from build123d import *

# Parameters (mm, degrees)
SKETCH1_W           = 40
SKETCH1_H           = 16
BOSS_EXTRUDE1_DEPTH = 1.5
SKETCH2_R           = 1.7
CUT_EXTRUDE1_DEPTH  = 22.592822882
SKETCH3_W           = 0.9
SKETCH3_H           = 0.4
CUT_EXTRUDE2_DEPTH  = 22.592822882
SKETCH5_R           = 1.65
CUT_EXTRUDE4_DEPTH  = 22.592822882
CUT_EXTRUDE5_DEPTH  = 0.05


with BuildPart() as part:
    # Sketch1 → Boss-Extrude1 (new body)
    with BuildSketch(Plane(origin=(0, 0, 0), x_dir=(1, 0, 0), z_dir=(0, 1, 0))):
        Rectangle(SKETCH1_W, SKETCH1_H)
    extrude(amount=BOSS_EXTRUDE1_DEPTH)

    # Sketch2 → Cut-Extrude1 (cut, through all)
    with BuildSketch(Plane(origin=(0, 1.5, 0), x_dir=(1, 0, 0), z_dir=(0, 1, 0))):
        with Locations(Location((0, 5.5, 0), (0, 0, 270))):
            Circle(SKETCH2_R)
        with Locations(Location((17.5, 5.5, 0), (0, 0, 270))):
            Circle(SKETCH2_R)
    extrude(amount=-CUT_EXTRUDE1_DEPTH, mode=Mode.SUBTRACT)

    # Sketch3 → Cut-Extrude2 (cut, through all)
    with BuildSketch(Plane(origin=(0, 1.5, 0), x_dir=(1, 0, 0), z_dir=(0, 1, 0))):
        with Locations((15.35, 1.3)):
            Rectangle(SKETCH3_W, SKETCH3_H)
        with Locations((5.15, 1.3)):
            Rectangle(SKETCH3_W, SKETCH3_H)
        with Locations((10.25, 1.3)):
            Rectangle(SKETCH3_W, SKETCH3_H)
    extrude(amount=-CUT_EXTRUDE2_DEPTH, mode=Mode.SUBTRACT)

    # Sketch5 → Cut-Extrude4 (cut, through all)
    with BuildSketch(Plane(origin=(0, 1.5, 0), x_dir=(1, 0, 0), z_dir=(0, 1, 0))):
        with Locations(Location((-15.78, 3.87, 0), (0, 0, 270))):
            Circle(SKETCH5_R)
        with Locations(Location((-15.78, -3.87, 0), (0, 0, 270))):
            Circle(SKETCH5_R)
    extrude(amount=-CUT_EXTRUDE4_DEPTH, mode=Mode.SUBTRACT)

    # Sketch6 → Cut-Extrude5 (cut)
    with BuildSketch(Plane(origin=(0, 1.5, 0), x_dir=(1, 0, 0), z_dir=(0, 1, 0))):
        Polygon((4.9, 1.5), (4.9, 2), (0.5208, 2), (0.5208, -2.8575), (-5.9792, -2.8575), (-5.9792, -2.2225), (-0.1192, -2.2225), (-0.1192, 2.5), (5.4, 2.5), (5.4, 1.5), align=None)
        Polygon((-5.9792, 2.8575), (-5.9792, 2.2225), (-0.4792, 2.2225), (-0.4792, 3), (15.1, 3), (15.1, 1.5), (15.6, 1.5), (15.6, 3.5), (-1.1192, 3.5), (-1.1192, 2.8575), align=None)
    extrude(amount=-CUT_EXTRUDE5_DEPTH, mode=Mode.SUBTRACT)


solid = part.part
Part model, mm, in its own coordinate system. A direction names the side the tool comes from. Round coordinates to 2 decimals unless told otherwise and drop trailing zeros. Write each loop counter-clockwise with the first axis right and the second up, starting at its lowest first coordinate (ties: lowest second). Pieces come first, ordered by that corner, then holes. Notation, with made-up numbers: M 59.5,-8.5 L 82.5,-8.5 A31 cw 82.5,30.5 Z; hole C 46.25,-23.75 d3. An arc over 180 degrees is marked long. Return JSON: item names as keys, results as strings. Group by question number.
(1) Two-plate mould, pull along X, no slides. Class faces 1 (the face through (0, 1, 8)), 2 (the face through (15.3, 0.8, -1.1)), 3 (the face through (-20, 1, 0)): +X half, -X half, draft (parallel to the pull), parting line (faces both ways), or undercut.
(2) Which spindle directions (+Z, -Z, +X, -X, +Y, -Y) get a long thin tool onto all of the face, cutting with end or side? Do faces 4 (the face through (5, 1, -1.5)), 5 (the face through (20, 1, 0)). Say none if no direction does.
(3) Saw through at B-B on y = 0.35. Write the cut outline in (x, z), then the cut area to 3 significant figures.
(4) Saw through at A-A on x = 17.5. Write the cut outline in (y, z).
(5) Saw through at D-D on x = -15.78. Write the cut outline in (y, z), then the cut area to 3 significant figures.
(6) Drill centre lines: probe 1 along X at (y, z) = (0.6, 3.75); probe 2 along X at (y, z) = (0.9, -4); probe 3 along Z at (x, y) = (17, 0.5). Where is each one in solid material? Low to high.
(7) Saw through at C-C on z = 3.87. Write the cut outline in (x, y), then the cut area to 4 significant figures.
Returned:
{
 "1": {"face 1": "draft", "face 2": "undercut", "face 3": "-X half"},
 "2": {"face 4": "+Y, -Y", "face 5": "+Z, -Z, +X, +Y, -Y"},
 "3": {"outline": "M -20,-8 L 20,-8 L 20,8 L -20,8 Z; hole C -15.78,-3.87 d3.3; hole C -15.78,3.87 d3.3; hole C 0,-5.5 d3.4; hole M 4.7,-1.5 L 5.6,-1.5 L 5.6,-1.1 L 4.7,-1.1 Z; hole M 9.8,-1.5 L 10.7,-1.5 L 10.7,-1.1 L 9.8,-1.1 Z; hole M 14.9,-1.5 L 15.8,-1.5 L 15.8,-1.1 L 14.9,-1.1 Z; hole C 17.5,-5.5 d3.4", "area": "604 mm²"},
 "4": {"outline": "M 0,-8 L 1.5,-8 L 1.5,-7.2 L 0,-7.2 Z; M 0,-3.8 L 1.5,-3.8 L 1.5,8 L 0,8 Z"},
 "5": {"outline": "M 0,-8 L 1.5,-8 L 1.5,-5.52 L 0,-5.52 Z; M 0,-2.22 L 1.5,-2.22 L 1.5,2.22 L 0,2.22 Z; M 0,5.52 L 1.5,5.52 L 1.5,8 L 0,8 Z", "area": "14.1 mm²"},
 "6": {"probe 1": "-20 to -17.43, -14.13 to 20", "probe 2": "-20 to -17.42, -14.14 to -0.8, 0.8 to 16.7, 18.3 to 20", "probe 3": "-8 to -7.12, -3.88 to 8"},
 "7": {"outline": "M -20,0 L -17.43,0 L -17.43,1.5 L -20,1.5 Z; M -14.13,0 L 20,0 L 20,1.5 L -14.13,1.5 Z", "area": "55.05 mm²"}
}
